Input: part model. Units: mm. Frame: model coordinates. Coordinates: 2 decimals unless noted, no trailing zeros. Write each loop counter-clockwise with the first axis right and the second up, starting at its lowest first coordinate (ties: lowest second). Pieces come first, ordered by that corner, then holes.
1) Pin query (flat end, axial travel): pin 1 Ø4 at (x, z) = (17.5, -4.5) entering from -Y; pin 2 Ø1.5 at (y, z) = (4, 4.5) entering from +X; pin 3 Ø2 at (y, z) = (3.5, -1.5) entering from +X. Return the tip coordinate at first contact, or that it passes through.
2) Draft query along Z for faces 1 (the cylindrical face through (10.174, 2.461, 4.732)), 2 (the flat face through (25.4, 0, 0)), 3 (the cylindrical face through (10.174, -1.294, 5.827)). Return one class per face: pulls with the +Z half, pulls with the -Z half, needs draft (parallel to the pull), parting line crosses it, or undercut.
3) Line query: L1, parallel to Z at x = 5.5, y = 0; L2, parallel to X at y = 0, z = 1.25; L3, parallel to Z at x = 22, y = 3. Output: solid intervals per line, ascending.
4) Section query A-A (x = 7.5). Output: boundary loops of the cut face in (y, z), then the cut area to 3 significant figures.
Autodesk Inventor part; units mm, degrees
ref_plane "YZ Plane" through (0, 0, 0) normal (1, 0, 0) x (0, 1, 0)
ref_plane "XZ Plane" through (0, 0, 0) normal (0, 1, 0) x (-1, 0, 0)
ref_plane "XY Plane" through (0, 0, 0) normal (0, 0, 1) x (1, 0, 0)
sketch "Sketch1" plane through (0, 0, 0) normal (1, 0, 0) x (0, 1, 0)
  circle A0 centre (0, 0) radius 5.969
  dimension "d0" = 11.938
extrude "Extrusion1" add sketch "Sketch1" along normal blind 25.4
fillet "Fillet1" radius 4.7625 1 edges at (25.4, -5.969, 0)
shell "Shell1" thickness 0.635 removed faces 1 at (0, -1.9689, -1.3194)
properties part number "piston cup" material "Glass"
Answer:
1. pin 1: stops at y = -5.42
1. pin 2: stops at x = 23.12
1. pin 3: stops at x = 25.12
2. face 1: undercut
2. face 2: needs draft
2. face 3: parting line crosses it
3. L1: z = -5.97 to -5.33, 5.33 to 5.97
3. L2: x = 24.76 to 25.4
3. L3: z = -4.93 to -4.13, 4.13 to 4.93
4. outline: circle Ø11.94 at (0, 0); hole circle Ø10.67 at (0, 0)
4. area: 22.5 mm2
